Can you work these out from the drawing? Everything is in mm from the part's minimum corner. A direction names the side the tool comes from. Coordinates: 2 decimals unless noted, no trailing zeros. Order: outer loops, then holes, each group sorted by start corner. A loop starts at its lowest first (then second) coordinate and runs counter-clockwise, first axis right, second up. Notation, with made-up numbers: (-27.75, 61) - (6.25, 61) arc R19 cw to (6.25, 76) - close; hole circle Ø1 at (59, 58). An arc over 180 degrees is marked (long way). Use a Markdown table: item, result. Add a question column.
(1) We'd pull the mould along Z, two halves only. Please class the marked faces 1, 2, 3 and 4: pulls with the +Z half, pulls with the -Z half, needs draft (parallel to the pull), parting line crosses it, or undercut.
(2) For pin 1 Ø3 at (y, z) = (4, 13) entering from +X; pin 2 Ø1.4 at (x, y) = (12, 3.5) entering from -Z; pin 3 Ø1.5 at (x, y) = (6.5, 1.5) entering from -Z, each with a flat end and sliding along its axis, tell me the tip position at first contact or that it passes through.
(3) If I drill on L1, parallel to X at y = 1.35, z = 12.25 (1 decimal); L2, parallel to Z at x = 13.25, y = 4.35; L3, parallel to X at y = 5.5, z = 10.5, over which ranges is the centre line in solid material (lowest first)? Write a range as [from, to].
(4) I want a section at B-B (y = 1.8). List the corners of the cut face in (x, z) for me.
(5) I want a section at D-D (x = 2.25). List the corners of the cut face in (y, z) for me.
(6) On a 3-axis mill with a long thin cutter (end or side, diameter ignored), from which of +Z, -Z, +X, -X, +Y, -Y can I reach the whole of each face in a straight line? I mean the marked faces 5 and 6. Say none if no direction works.
(7) I want a section at C-C (z = 18.5). List the corners of the cut face in (x, y) for me (1 decimal).
(8) I want a section at A-A (x = 11). List the corners of the cut face in (y, z) for me, and give its area (3 significant figures).
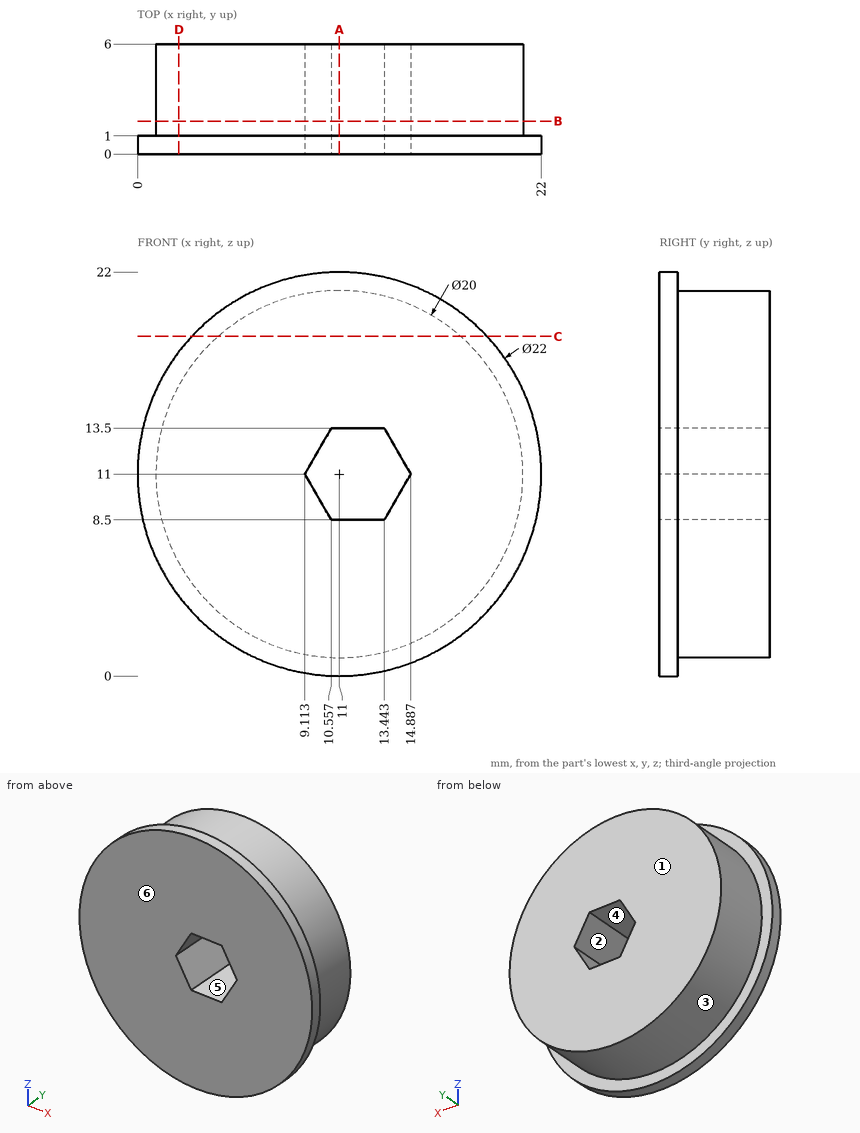
Answers follow:
| question | item | result |
|---|---|---|
| 1 | face 1 | needs draft |
| 1 | face 2 | undercut |
| 1 | face 3 | parting line crosses it |
| 1 | face 4 | undercut |
| 2 | pin 1 | stops at x = 20.99 |
| 2 | pin 2 | stops at z = 1 |
| 2 | pin 3 | stops at z = 0.73 |
| 3 | L1 | x = [1.1, 9.8], [14.2, 20.9] |
| 3 | L2 | z = [1.26, 8.5], [13.5, 20.74] |
| 3 | L3 | x = [1.01, 9.4], [14.6, 20.99] |
| 4 | outline | circle Ø20 at (11, 11); hole (9.11, 11) - (10.56, 8.5) - (13.44, 8.5) - (14.89, 11) - (13.44, 13.5) - (10.56, 13.5) - close |
| 5 | outline | (0, 4.33) - (1, 4.33) - (1, 6.16) - (6, 6.16) - (6, 15.84) - (1, 15.84) - (1, 17.67) - (0, 17.67) - close |
| 6 | face 5 | +Y, -Y |
| 6 | face 6 | +Z, -Z, +X, -X, -Y |
| 7 | outline | (3, 0) - (19, 0) - (19, 1) - (17.6, 1) - (17.6, 6) - (4.4, 6) - (4.4, 1) - (3, 1) - close |
| 8 | outline | (0, 0) - (1, 0) - (1, 1) - (6, 1) - (6, 8.5) - (0, 8.5) - close; (0, 13.5) - (6, 13.5) - (6, 21) - (1, 21) - (1, 22) - (0, 22) - close |
| 8 | area | 92.0 mm² |
